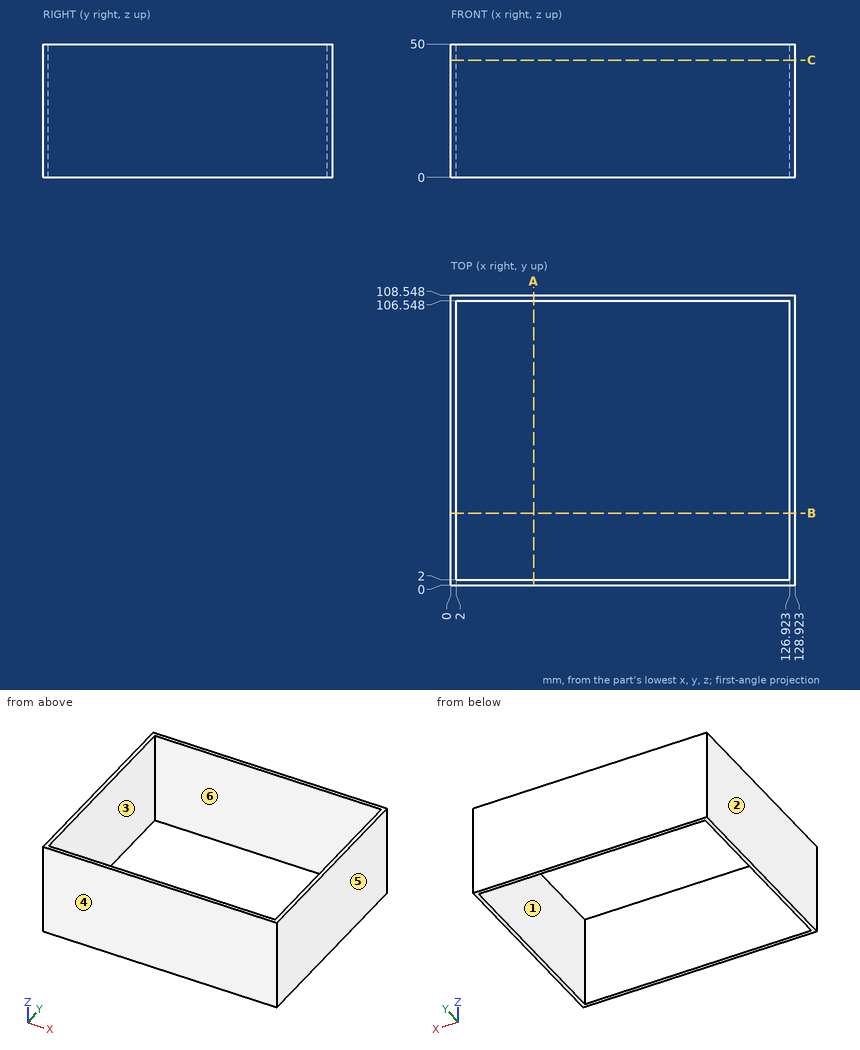
Check sheet for the drawn part. Datum: minimum x, y, z corner. Units: mm. A direction names the side the tool comes from. Round coordinates to 2 decimals unless told otherwise and drop trailing zeros. Order: outer loops, then holes, each group sorted by start corner. A loop starts at its lowest first (then second) coordinate and runs counter-clockwise, first axis right, second up. Notation, with made-up numbers: M 52.5,-22.75 L 65.5,-22.75 A6 ccw 65.5,-17.75 Z; hole C 37.25,72 d6. An arc over 180 degrees is marked long. Answer in a Markdown table with one row per item.
(1) Material ranges on line 1 along X through (y, z) = (99.5, 35); line 2 along Y through (x, z) = (71, 45), recorded low to high. Write a range as from..to.
Findings:
| item | result |
|---|---|
| line 1 | x = 0..2, 126.92..128.92 |
| line 2 | y = 0..2, 106.55..108.55 |
(2) Section check B-B on y = 27. Record the boundary of the cut face in (x, z), plus the area to 3 significant figures.
Findings:
| item | result |
|---|---|
| outline | M 0,0 L 2,0 L 2,50 L 0,50 Z; M 126.92,0 L 128.92,0 L 128.92,50 L 126.92,50 Z |
| area | 200 mm^2 |
(3) Set-up check for the marked faces 5 and 6: record each of +Z, -Z, +X, -X, +Y, -Y from which the full face is reachable in a straight line by a thin tool's end or side.
Findings:
| item | result |
|---|---|
| face 5 | +Z, -Z, +X, +Y, -Y |
| face 6 | +Z, -Z |
(4) Draft check along Y on the marked faces 1, 2, 3 and 4. Enter one of: +Y half, -Y half, draft (parallel to the pull), parting line (faces both ways), or undercut.
Findings:
| item | result |
|---|---|
| face 1 | undercut |
| face 2 | draft |
| face 3 | undercut |
| face 4 | -Y half |
(5) Section check A-A on x = 31. Record the boundary of the cut face in (y, z), plus the area to 3 significant figures.
Findings:
| item | result |
|---|---|
| outline | M 0,0 L 2,0 L 2,50 L 0,50 Z; M 106.55,0 L 108.55,0 L 108.55,50 L 106.55,50 Z |
| area | 200 mm^2 |
(6) Section check C-C on z = 44. Record the boundary of the cut face in (x, y).
Findings:
| item | result |
|---|---|
| outline | M 0,0 L 128.92,0 L 128.92,108.55 L 0,108.55 Z; hole M 2,2 L 126.92,2 L 126.92,106.55 L 2,106.55 Z |
